Check sheet for the modelled part. Datum: model origin and axes. Units: mm. Face numbers are marked on the shaded views. A direction names the side the tool comes from. Coordinates: 2 decimals unless noted, no trailing zeros. Write each loop counter-clockwise with the first axis right and the second up, starting at its lowest first coordinate (ties: lowest second). Pieces come first, ordered by that corner, then holes. Notation, with made-up numbers: M 47.25,49 L 72.25,49 A26 cw 72.25,72 Z; hole C 82.5,70 d5. An arc over 180 degrees is marked long. Answer as CSV lines item,"result".
from build123d import *

# Parameters (mm, degrees)
SKETCH2_R           = 8
BOSS_EXTRUDE1_DEPTH = 2
FILLET1_R           = 0.5
SKETCH3_R           = 1.6
CUT_EXTRUDE1_DEPTH  = 10
SKETCH4_R           = 4
CUT_EXTRUDE2_DEPTH  = 10
SKETCH5_R           = 8
CUT_EXTRUDE3_DEPTH  = 3


with BuildPart() as part:
    # Sketch1 → Revolve1 (revolve)
    with BuildSketch(Plane.XY):
        Polygon((0, 0), (0, 20.292893219), (0.707106781, 21), (5.9, 21), (5.9, 0), align=None)
    revolve(axis=Axis((0, 0, 0), (1, 0, 0)))

    # Sketch2 → Boss-Extrude1 (add)
    with BuildSketch(Plane.ZY):
        with BuildLine():
            Line((-11.5, -4.898979486), (-11.5, 4.898979486))
            ThreePointArc((-11.5, 4.898979486), (0, 12.5), (11.5, 4.898979486))
            Line((11.5, 4.898979486), (11.5, -4.898979486))
            ThreePointArc((11.5, -4.898979486), (0, -12.5), (-11.5, -4.898979486))
        make_face()
        Circle(SKETCH2_R, mode=Mode.SUBTRACT)
    extrude(amount=BOSS_EXTRUDE1_DEPTH)

    # Fillet1
    fillet1_edges = [part.edges().sort_by_distance(p)[0] for p in [
        (-2, 12.5, 0),
        (-2, 0, -11.5),
        (-2, -12.5, 0),
        (-2, 0, 11.5),
        (0, 12.5, 0),
        (-1, 4.898979486, 11.5),
        (0, 0, -11.5),
        (-1, 4.898979486, -11.5),
        (0, -12.5, 0),
        (-1, -4.898979486, -11.5),
        (0, 0, 11.5),
        (-1, -4.898979486, 11.5),
        (-2, 0, -8),
    ]]
    fillet(fillet1_edges, radius=FILLET1_R)

    # Sketch3 → Cut-Extrude1 (cut)
    with BuildSketch(Plane.ZY):
        with Locations((12.374368671, 12.374368671)):
            Circle(SKETCH3_R)
        with Locations((-12.374368671, 12.374368671)):
            Circle(SKETCH3_R)
        with Locations((-12.374368671, -12.374368671)):
            Circle(SKETCH3_R)
        with Locations((12.374368671, -12.374368671)):
            Circle(SKETCH3_R)
    extrude(amount=-CUT_EXTRUDE1_DEPTH, mode=Mode.SUBTRACT)

    # Sketch4 → Cut-Extrude2 (cut)
    with BuildSketch(Plane.ZY):
        Circle(SKETCH4_R)
    extrude(amount=-CUT_EXTRUDE2_DEPTH, mode=Mode.SUBTRACT)

    # Sketch5 → Cut-Extrude3 (cut)
    with BuildSketch(Plane.ZY):
        Circle(SKETCH5_R)
    extrude(amount=-CUT_EXTRUDE3_DEPTH, mode=Mode.SUBTRACT)


solid = part.part
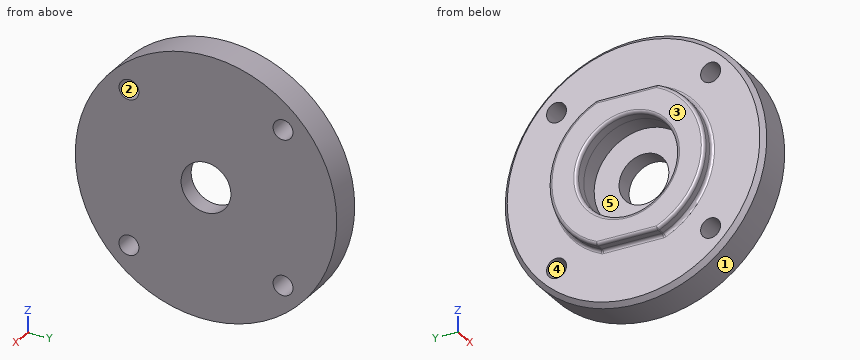
1) Section check C-C, the plane x = 1.5. Record the boundary of the cut face in (y, z), plus the area to 3 significant figures.
Answer key:
outline,"C 0,0 d42; hole C -12.37,-12.37 d3.2; hole C -12.37,12.37 d3.2; hole C 0,0 d16; hole C 12.37,-12.37 d3.2; hole C 12.37,12.37 d3.2"
area,"1,150 mm2"
2) Section check A-A, the plane y = 0. Record the boundary of the cut face in (x, z).
Answer key:
outline,"M -2,-11 A0.5 ccw -1.5,-11.5 L -0.5,-11.5 A0.5 cw 0,-12 L 0,-20.29 L 0.71,-21 L 5.9,-21 L 5.9,-4 L 3,-4 L 3,-8 L -1.5,-8 A0.5 ccw -2,-8.5 Z; M -2,8.5 A0.5 ccw -1.5,8 L 3,8 L 3,4 L 5.9,4 L 5.9,21 L 0.71,21 L 0,20.29 L 0,12 A0.5 cw -0.5,11.5 L -1.5,11.5 A0.5 ccw -2,11 Z"
3) Section check D-D, the plane z = -12.5. Give the number of separate pieces and of enclosed holes in the cut face, plus the area to 3 significant figures.
Answer key:
separate pieces,"3"
enclosed holes,"0"
area,"161 mm2"
4) Thickness scan on line 1 along Z through (x, y) = (2.5, 11); line 2 along Z through (x, y) = (5, 12); line 3 along X through (y, z) = (-15.5, 5). Record the ranges inside material, lowest first.
Answer key:
line 1,"z = -17.89 to -13.19, -11.56 to 11.56, 13.19 to 17.89"
line 2,"z = -17.23 to -13.93, -10.82 to 10.82, 13.93 to 17.23"
line 3,"x = 0 to 5.9"
5) Section check B-B, the plane z = 0. Record the boundary of the cut face in (x, y).
Answer key:
outline,"M -2,-12 A0.5 ccw -1.5,-12.5 L -0.5,-12.5 A0.5 cw 0,-13 L 0,-20.29 L 0.71,-21 L 5.9,-21 L 5.9,-4 L 3,-4 L 3,-8 L -1.5,-8 A0.5 ccw -2,-8.5 Z; M -2,8.5 A0.5 ccw -1.5,8 L 3,8 L 3,4 L 5.9,4 L 5.9,21 L 0.71,21 L 0,20.29 L 0,13 A0.5 cw -0.5,12.5 L -1.5,12.5 A0.5 ccw -2,12 Z"
6) Tool access check on the marked faces 4 and 5. Record the directions out of +Z, -Z, +X, -X, +Y, -Y that give a thin tool (end or side, any length) a straight path to the whole face; none if there is none.
Answer key:
face 4,"+X, -X"
face 5,"-X"
7) Mould release check, pull along Y, two halves, no side actions. Record for the marked faces 1, 2 and 3: pulls with the +Y half, pulls with the -Y half, needs draft (parallel to the pull), parting line crosses it, or undercut.
Answer key:
face 1,"parting line crosses it"
face 2,"undercut"
face 3,"needs draft"
8) Depth check by flat-ended pin: P1, Ø5, axis at y = 2.5, z = -4, coming from the -X side; P2, Ø5, axis at y = -12.37, z = -12.37, coming from the -X side; P3, Ø1, axis at x = 3.5, y = 15, coming from the -Z side. Enter the tip coordinate at first touch or a pass-through.
Answer key:
P1,"stops at x = 3"
P2,"stops at x = 0"
P3,"stops at z = -15.19"
